```python
from build123d import *

# Parameters (mm, degrees)
F2_SIZE = 5
F3_R    = 2


with BuildPart() as f1:
    # F0 (on Front) → F1 (revolve)
    with BuildSketch(Plane.XZ):
        Polygon((5.7735026919, 0), (-5.7735026919, 0), (-11.5470053838, -10), (-5.7735026919, -20), (5.7735026919, -20), (11.5470053838, -10), align=None)
    revolve(axis=Axis((0, 0, -20), (-1, 0, 0)))

    # F2
    f2_edges = [f1.edges().sort_by_distance(p)[0] for p in [
        (5.773503, 0, -40),
        (-5.773503, 0, -40),
        (0, 0, 0),
    ]]
    chamfer(f2_edges, length=F2_SIZE)

    # F3
    f3_edges = [f1.edges().sort_by_distance(p)[0] for p in [
        (-11.547005, 0, -30),
        (-8.273503, 0, -35.669869),
        (-0.773503, 0, -39.999995),
        (0.773503, 0, -39.999995),
        (8.273503, 0, -35.669869),
        (11.547005, 0, -30),
        (8.660254, 0, -15),
    ]]
    fillet(f3_edges, radius=F3_R)


solid = f1.part
```
Verification items for the finished model (mm, model axes). Round coordinates to 2 decimals unless told otherwise and drop trailing zeros.
1. Scan lines: L1, parallel to Y at x = -9.5, z = -24; L2, parallel to Z at x = 10, y = -2.5; L3, parallel to X at y = 4.5, z = -11. Record each from-to range of solid material in increasing order.
2. Draft check along Z on faces 1 (the cylindrical face through (-0.003, 6.007, -0.924)), 2 (the conical face through (-6.6, -0.6, -18.7)). Enter one of: +Z half, -Z half, draft (parallel to the pull), parting line (faces both ways), or undercut.
3. Gauge pin test, flat ends, axial feed: P1, Ø1, axis at y = 1, z = -9, coming from the -X side; P2, Ø2, axis at y = -12.5, z = -10.5, coming from the +X side; P3, Ø4, axis at y = 6.5, z = -22, coming from the -X side. Record the tip position at first contact, or that the pin passes through.
Answer:
1. L1: y = -12.94 to -5.07, 5.07 to 12.94
1. L2: z = -32.43 to -26.88, -13.12 to -7.57
1. L3: x = -11.24 to 11.24
2. face 1: parting line
2. face 2: undercut
3. P1: stops at x = -11.16
3. P2: stops at x = 8.83
3. P3: stops at x = -10.85
